Autodesk Inventor part; units mm, degrees
ref_plane "YZ Plane" through (0, 0, 0) normal (1, 0, 0) x (0, 1, 0)
ref_plane "XZ Plane" through (0, 0, 0) normal (0, 1, 0) x (-1, 0, 0)
ref_plane "XY Plane" through (0, 0, 0) normal (0, 0, 1) x (1, 0, 0)
sketch "Sketch1" plane through (0, 0, 0) normal (0, 0, 1) x (1, 0, 0)
  line L0 (0, 0) -> (-200, 0)
  line L1 (-200, 0) -> (-200, 60)
  line L2 (-200, 60) -> (0, 60)
  line L3 (0, 60) -> (0, 0)
  dimension "d0" = 200
  dimension "d1" = 60
extrude "Extrusion1" add sketch "Sketch1" along normal blind 40
sketch "Sketch2" plane through (0, 0, 40) normal (0, 0, 1) x (1, 0, 0)
  circle A0 centre (-25, 30) radius 20
  line L0 (0, 60) -> (-200, 60)
  line L1 (0, 0) -> (0, 60)
  dimension "d4" = 40
  dimension "d5" = 30
  dimension "d6" = 25
extrude "Extrusion2" add sketch "Sketch2" along normal mid plane 40
sketch "Sketch3" plane through (0, 0, 0) normal (0, 0, -1) x (-1, 0, 0)
  circle A0 centre (25, 30) radius 20
  circle A1 centre (25, 30) radius 20
  point P0 (0, 0)
extrude "Extrusion3" add sketch "Sketch3" along normal mid plane 40
sketch "Sketch4" plane through (-200, 0, 0) normal (-1, 0, 0) x (0, 0, 1)
  line L0 (0, 60) -> (40, 60)
  line L1 (25, 0) -> (15, 0)
  line L2 (15, 0) -> (15, 60)
  line L3 (15, 60) -> (25, 60)
  line L4 (25, 60) -> (25, 0)
  line L5 (0, 60) -> (0, 0)
  line L6 (40, 60) -> (40, 0)
  dimension "d11" = 10
  dimension "d12" = 60
  dimension "d13" = 15
  dimension "d14" = 15
  dimension "d15" = 60
extrude "Extrusion4" add sketch "Sketch4" along normal mid plane 50
fillet "Fillet1" radius 30 2 edges at (-200, 30, 0) (-200, 30, 40)
fillet "Fillet2" radius 5 2 edges at (-225, 60, 20) (-225, 0, 20)
properties part number "Part4final"
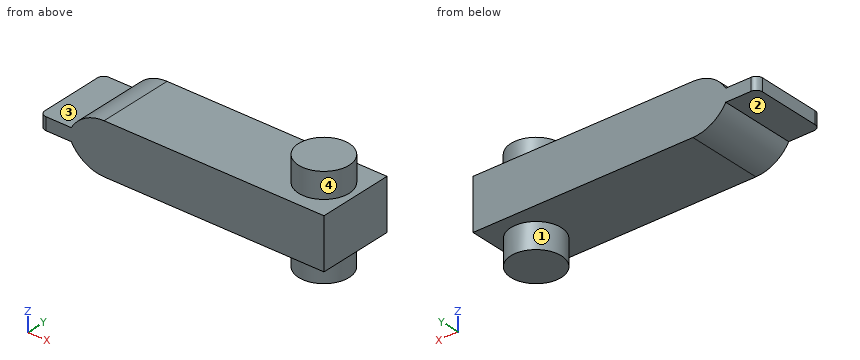
CAD build for the part. Positions are in the model's coordinates, mm. Face numbers are marked on the shaded views. A direction names the side the tool comes from. Give positions to 0.01 mm unless a question says otherwise; leave off trailing zeros. Loops run counter-clockwise (first coordinate to the right, second up) from the corner with the lowest first, then second, coordinate; pieces in that order, holes last. Notation, with made-up numbers: (35, 64) -> (74, 64) arc R18 cw to (74, 84) -> close; hole circle Ø3 at (66.25, 11). An arc over 180 degrees is marked (long way). Use a Markdown table: item, result.
1. Slice it at B-B (y = 30). List the corners of the cut face in (x, z), plus the area to 3 significant figures.
Check result:
| item | result |
|---|---|
| outline | (-225, 15) -> (-200, 15) arc R30 ccw to (-174.02, 0) -> (-45, 0) -> (-45, -20) -> (-5, -20) -> (-5, 0) -> (0, 0) -> (0, 40) -> (-5, 40) -> (-5, 60) -> (-45, 60) -> (-45, 40) -> (-174.02, 40) arc R30 ccw to (-200, 25) -> (-225, 25) -> close |
| area | 9,620 mm^2 |
2. Slice it at C-C (z = 47.5). List the corners of the cut face in (x, y).
Check result:
| item | result |
|---|---|
| outline | circle Ø40 at (-25, 30) |
3. Flat gauge pins, fed straight in: pin 1 (3 mm diameter, centred on y = 20, z = 24, fed in from +X); pin 2 (18 mm diameter, centred on x = -67.5, y = 16.5, fed in from -Z); pin 3 (1.5 mm diameter, centred on y = 36, z = 51.5, fed in from +X); pin 4 (4 mm diameter, centred on x = -192, y = 24, fed in from +Z). Where does each tip first touch, or does it go through?
Check result:
| item | result |
|---|---|
| pin 1 | stops at x = 0 |
| pin 2 | stops at z = 0 |
| pin 3 | stops at x = -5.7 |
| pin 4 | stops at z = 35.39 |
4. Which spindle directions (+Z, -Z, +X, -X, +Y, -Y) get a long thin tool onto all of the face, cutting with end or side? Do the marked faces 1, 2, 3 and 4. Say none if no direction does.
Check result:
| item | result |
|---|---|
| face 1 | -Z |
| face 2 | -Z, -X, +Y, -Y |
| face 3 | +Z, -X, +Y, -Y |
| face 4 | +Z |
5. Wall check: L1, parallel to Z at x = -162, y = 27.5; L2, parallel to Z at x = -178.5, y = 48; L3, parallel to Y at x = -22.5, z = 43.5. Give the ranges that are in metal, low to high. Write a range as [from, to].
Check result:
| item | result |
|---|---|
| L1 | z = [0, 40] |
| L2 | z = [0.34, 39.66] |
| L3 | y = [10.16, 49.84] |
6. Slice it at D-D (y = 42). List the corners of the cut face in (x, z), plus the area to 3 significant figures.
Check result:
| item | result |
|---|---|
| outline | (-225, 15) -> (-200, 15) arc R30 ccw to (-174.02, 0) -> (-41, 0) -> (-41, -20) -> (-9, -20) -> (-9, 0) -> (0, 0) -> (0, 40) -> (-9, 40) -> (-9, 60) -> (-41, 60) -> (-41, 40) -> (-174.02, 40) arc R30 ccw to (-200, 25) -> (-225, 25) -> close |
| area | 9,300 mm^2 |
7. Slice it at A-A (x = -25). List the corners of the cut face in (y, z), plus the area to 3 significant figures.
Check result:
| item | result |
|---|---|
| outline | (0, 0) -> (10, 0) -> (10, -20) -> (50, -20) -> (50, 0) -> (60, 0) -> (60, 40) -> (50, 40) -> (50, 60) -> (10, 60) -> (10, 40) -> (0, 40) -> close |
| area | 4,000 mm^2 |
